```python
from build123d import *

# Parameters (mm, degrees)
SKETCH_1_W                   = 34
SKETCH_1_H                   = 34
SKETCH_1_R                   = 2.25
EXTRUDE_1_DEPTH              = 10
SKETCH_1_3_W                 = 30
SKETCH_1_3_H                 = 30
CUT_EXTRUDE_1_DEPTH          = 6
CHAMFER_1_SIZE               = 2
HOLE_WIZARD_M2_1_D           = 2.2
HOLE_WIZARD_M2_1_CBORE_D     = 4.3
HOLE_WIZARD_M2_1_CBORE_DEPTH = 2.3


with BuildPart() as part:
    # Sketch 1 → Extrude 1 (new body)
    with BuildSketch(Plane(origin=(0, 0, 0), x_dir=(1, 0, 0), z_dir=(0, 1, 0))):
        Rectangle(SKETCH_1_W, SKETCH_1_H)
        with Locations(Location((0, 0, 0), (0, 0, 270))):
            Circle(SKETCH_1_R, mode=Mode.SUBTRACT)
    extrude(amount=EXTRUDE_1_DEPTH)

    # Sketch 1_3 → Cut-Extrude 1 (cut)
    with BuildSketch(Plane(origin=(0, 0, 0), x_dir=(1, 0, 0), z_dir=(0, 1, 0))):
        Rectangle(SKETCH_1_3_W, SKETCH_1_3_H)
    extrude(amount=CUT_EXTRUDE_1_DEPTH, mode=Mode.SUBTRACT)

    # Chamfer 1
    chamfer_1_edges = [part.edges().sort_by_distance(p)[0] for p in [
        (-15, 3, 15),
        (15, 3, 15),
        (15, 3, -15),
        (-15, 3, -15),
        (-17, 5, 17),
        (17, 5, 17),
        (17, 5, -17),
        (-17, 5, -17),
    ]]
    chamfer(chamfer_1_edges, length=CHAMFER_1_SIZE)

    # Hole Wizard M2 _1 (through all)
    with Locations(Plane(origin=(0, 6, 0), x_dir=(-1, 0, 0), z_dir=(0, -1, 0))):
        with Locations((0, 6.25), (6.25, 0), (0, -6.25), (-6.25, 0)):
            CounterBoreHole(HOLE_WIZARD_M2_1_D / 2, HOLE_WIZARD_M2_1_CBORE_D / 2, HOLE_WIZARD_M2_1_CBORE_DEPTH)


solid = part.part
```
Read the model definition and answer for the solid it produces. Units are mm, in the model's axes. A direction names the side the tool comes from. Coordinates: 2 decimals unless noted, no trailing zeros. Loops run counter-clockwise (first coordinate to the right, second up) from the corner with the lowest first, then second, coordinate; pieces in that order, holes last.
(1) The part is cut by section D-D (y = 1.5). Determine the outline of the cut face in (x, z).
Solution:
outline: (-17, -15) - (-15, -17) - (15, -17) - (17, -15) - (17, 15) - (15, 17) - (-15, 17) - (-17, 15) - close; hole (-15, -13) - (-13, -15) - (13, -15) - (15, -13) - (15, 13) - (13, 15) - (-13, 15) - (-15, 13) - close
(2) The mould has two halves that part along X. Classify faces 3 (the face through (0.59, 9.16, 5.32)), 4 (the face through (16, 5, -16)), 5 (the face through (-16, 5, 16)): released by +X, released by -X, zero draft, split by the parting line, or undercut.
Solution:
face 3: undercut
face 4: released by +X
face 5: released by -X
(3) The part is cut by section C-C (z = -9). Determine the outline of the cut face in (x, y).
Solution:
outline: (-17, 0) - (-15, 0) - (-15, 6) - (15, 6) - (15, 0) - (17, 0) - (17, 10) - (-17, 10) - close
(4) The part is cut by section A-A (x = 0). Determine the outline of the cut face in (y, z).
Solution:
outline: (0, -17) - (10, -17) - (10, -7.35) - (8.3, -7.35) - (8.3, -8.4) - (6, -8.4) - (6, -15) - (0, -15) - close; (0, 15) - (6, 15) - (6, 8.4) - (8.3, 8.4) - (8.3, 7.35) - (10, 7.35) - (10, 17) - (0, 17) - close; (6, -4.1) - (8.3, -4.1) - (8.3, -5.15) - (10, -5.15) - (10, -2.25) - (6, -2.25) - close; (6, 2.25) - (10, 2.25) - (10, 5.15) - (8.3, 5.15) - (8.3, 4.1) - (6, 4.1) - close
(5) The part is cut by section B-B (x = -6.25). Determine the outline of the cut face in (y, z), and give its area (3 significant figures).
Solution:
outline: (0, -17) - (10, -17) - (10, -1.1) - (8.3, -1.1) - (8.3, -2.15) - (6, -2.15) - (6, -15) - (0, -15) - close; (0, 15) - (6, 15) - (6, 2.15) - (8.3, 2.15) - (8.3, 1.1) - (10, 1.1) - (10, 17) - (0, 17) - close
area: 146 mm2
(6) A tool of negligible diameter and unlimited length cuts with its end or side. For faces 1 (the face through (15, 3, 0)), 2 (the face through (0, 5, 17)), from which of +Z, -Z, +X, -X, +Y, -Y can it reach the whole face along a straight path? Write none if from no direction.
Solution:
face 1: -Y
face 2: +Z, +X, -X, +Y, -Y
(7) Flat-ended cylindrical pins translate along their axes: pin 1 Ø3.5 at (x, z) = (0, 0) entering from +Y; pin 2 Ø4.5 at (x, z) = (0.5, -5.5) entering from -Y; pin 3 Ø3.5 at (x, z) = (6.25, 0) entering from -Y. Find the tip coordinate at first contact, or state that the pin passes through.
Solution:
pin 1: passes through
pin 2: stops at y = 6
pin 3: stops at y = 8.3
(8) Consider line 1 along Z through (x, y) = (0, 9.15); line 2 along Z through (x, y) = (0, 7.65); line 3 along Z through (x, y) = (6.5, 4.75). Determine where each line is inside the solid, lowest interval first.
Solution:
line 1: z = -17 to -7.35, -5.15 to -2.25, 2.25 to 5.15, 7.35 to 17
line 2: z = -17 to -8.4, -4.1 to -2.25, 2.25 to 4.1, 8.4 to 17
line 3: z = -17 to -15, 15 to 17
